from build123d import *

# Parameters (mm, degrees)
BOSS_EXTRUDE1_DEPTH = 3.175
SKETCH2_R           = 4
SKETCH2_R_2         = 3
CUT_EXTRUDE1_DEPTH  = 1733.72226626


with BuildPart() as part:
    # Sketch1 → Boss-Extrude1 (new body)
    with BuildSketch(Plane.XY):
        with BuildLine():
            Line((66.635268781, 1721.56), (186.335268781, 1721.56))
            ThreePointArc((186.335268781, 1721.56), (193.406336593, 1718.631067812), (196.335268781, 1711.56))
            Line((196.335268781, 1711.56), (196.335268781, 1591.86))
            ThreePointArc((196.335268781, 1591.86), (193.406336593, 1584.788932188), (186.335268781, 1581.86))
            Line((186.335268781, 1581.86), (66.635268781, 1581.86))
            ThreePointArc((66.635268781, 1581.86), (59.564200969, 1584.788932188), (56.635268781, 1591.86))
            Line((56.635268781, 1591.86), (56.635268781, 1711.56))
            ThreePointArc((56.635268781, 1711.56), (59.564200969, 1718.631067812), (66.635268781, 1721.56))
        make_face()
    extrude(amount=BOSS_EXTRUDE1_DEPTH)

    # Sketch2 → Cut-Extrude1 (cut, through all)
    with BuildSketch(Plane(origin=(0, 0, 0), x_dir=(-1, 0, 0), z_dir=(0, 0, -1))):
        with Locations((-71.485268781, 1638.71)):
            Circle(SKETCH2_R)
        with Locations((-71.485268781, 1676.71)):
            Circle(SKETCH2_R)
        with Locations((-117.485268781, 1638.71)):
            Circle(SKETCH2_R)
        with Locations((-181.485268781, 1706.71)):
            Circle(SKETCH2_R_2)
        with Locations((-71.485268781, 1706.71)):
            Circle(SKETCH2_R_2)
        with Locations((-181.485268781, 1596.71)):
            Circle(SKETCH2_R_2)
        with Locations((-71.485268781, 1596.71)):
            Circle(SKETCH2_R_2)
    extrude(amount=-CUT_EXTRUDE1_DEPTH, mode=Mode.SUBTRACT)


solid = part.part
Here's how the part is built. I have some questions about the finished solid (model axes, mm). Round coordinates to 2 decimals unless told otherwise and drop trailing zeros. Write each loop counter-clockwise with the first axis right and the second up, starting at its lowest first coordinate (ties: lowest second). Pieces come first, ordered by that corner, then holes.
1. Suppose I cut it at C-C (x = 72.5). List the corners of the cut face in (y, z) for me (3 decimals).
2. Suppose I cut it at A-A (y = 1596.71). List the corners of the cut face in (x, z) for me (3 decimals).
3. Suppose I cut it at D-D (y = 1676.71). List the corners of the cut face in (x, z) for me (3 decimals).
4. I need wall thicknesses on L1, parallel to X at y = 1706.71, z = 1.7; L2, parallel to X at y = 1637.5, z = 1.9; L3, parallel to Y at x = 75, z = 2.95. Which ranges of each line are inside material? Lowest first, please.
5. If we mould it in two halves opening along X, with no side actions, what happens to faces 1 (the flat face through (56.635, 1651, 2)), 2 (the flat face through (127, 1653, 0)), 3 (the cylindrical face through (72.006, 1642.676, 1.565))? For each: released by +X, released by -X, zero draft, split by the parting line, or undercut.
6. Suppose I cut it at B-B (z = 1). List the corners of the cut face in (x, y) for me, and give its area (3 significant figures).
Answer sheet:
1. outline: (1581.86, 0) - (1593.887, 0) - (1593.887, 3.175) - (1581.86, 3.175) - close; (1599.533, 0) - (1634.841, 0) - (1634.841, 3.175) - (1599.533, 3.175) - close; (1642.579, 0) - (1672.841, 0) - (1672.841, 3.175) - (1642.579, 3.175) - close; (1680.579, 0) - (1703.887, 0) - (1703.887, 3.175) - (1680.579, 3.175) - close; (1709.533, 0) - (1721.56, 0) - (1721.56, 3.175) - (1709.533, 3.175) - close
2. outline: (56.635, 0) - (68.485, 0) - (68.485, 3.175) - (56.635, 3.175) - close; (74.485, 0) - (178.485, 0) - (178.485, 3.175) - (74.485, 3.175) - close; (184.485, 0) - (196.335, 0) - (196.335, 3.175) - (184.485, 3.175) - close
3. outline: (56.635, 0) - (67.485, 0) - (67.485, 3.175) - (56.635, 3.175) - close; (75.485, 0) - (196.335, 0) - (196.335, 3.175) - (75.485, 3.175) - close
4. L1: x = 56.64 to 68.49, 74.49 to 178.49, 184.49 to 196.34
4. L2: x = 56.64 to 67.67, 75.3 to 113.67, 121.3 to 196.34
4. L3: y = 1581.86 to 1636.8, 1640.62 to 1674.8, 1678.62 to 1721.56
5. face 1: released by -X
5. face 2: zero draft
5. face 3: undercut
6. outline: (56.64, 1591.86) arc R10 ccw to (66.64, 1581.86) - (186.34, 1581.86) arc R10 ccw to (196.34, 1591.86) - (196.34, 1711.56) arc R10 ccw to (186.34, 1721.56) - (66.64, 1721.56) arc R10 ccw to (56.64, 1711.56) - close; hole circle Ø8 at (71.49, 1638.71); hole circle Ø8 at (71.49, 1676.71); hole circle Ø6 at (71.49, 1596.71); hole circle Ø6 at (71.49, 1706.71); hole circle Ø8 at (117.49, 1638.71); hole circle Ø6 at (181.49, 1596.71); hole circle Ø6 at (181.49, 1706.71)
6. area: 19,200 mm2
